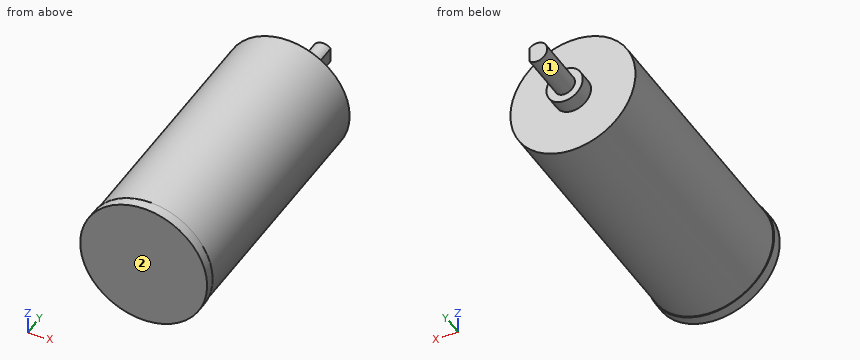
```python
from build123d import *

# Parameters (mm, degrees)
SKETCH_1_R      = 12.25
EXTRUDE_1_DEPTH = 2
SKETCH_2_R      = 12.075
EXTRUDE_2_DEPTH = 51.65
SKETCH_3_R      = 3.5
EXTRUDE_3_DEPTH = 3
EXTRUDE_4_DEPTH = 10


with BuildPart() as part:
    # Эскиз1 → Бобышка-Вытянуть1 (new body)
    with BuildSketch(Plane(origin=(0, 0, 0), x_dir=(1, 0, 0), z_dir=(0, 1, 0))):
        Circle(SKETCH_1_R)
    extrude(amount=EXTRUDE_1_DEPTH)

    # Эскиз2 → Бобышка-Вытянуть2 (add)
    with BuildSketch(Plane(origin=(0, 0, 0), x_dir=(1, 0, 0), z_dir=(0, 1, 0))):
        Circle(SKETCH_2_R)
    extrude(amount=EXTRUDE_2_DEPTH)

    # Эскиз3 → Бобышка-Вытянуть3 (add)
    with BuildSketch(Plane(origin=(0, 51.65, 0), x_dir=(1, 0, 0), z_dir=(0, 1, 0))):
        Circle(SKETCH_3_R)
    extrude(amount=EXTRUDE_3_DEPTH)

    # Эскиз4 → Бобышка-Вытянуть4 (add)
    with BuildSketch(Plane(origin=(0, 54.65, 0), x_dir=(1, 0, 0), z_dir=(0, 1, 0))):
        with BuildLine():
            Line((1.45, 0), (1.45, 1.377497731))
            ThreePointArc((1.45, 1.377497731), (-2, 0), (1.45, -1.377497731))
            Line((1.45, -1.377497731), (1.45, 0))
        make_face()
    extrude(amount=EXTRUDE_4_DEPTH)


solid = part.part
```
For this review, take the finished solid that the model builds, in its own axes (mm). Face numbers are marked on the shaded views. A direction names the side the tool comes from. Coordinates: 2 decimals unless noted, no trailing zeros. Write each loop counter-clockwise with the first axis right and the second up, starting at its lowest first coordinate (ties: lowest second). Pieces come first, ordered by that corner, then holes. Notation, with made-up numbers: (25, 1) - (34, 1) arc R23 ccw to (34, 22) - close; hole circle Ø6 at (37, 17). An arc over 180 degrees is marked (long way). Put each result on its own line as item: value.
1. Add section C-C, the plane y = 29. Give the boundary of the cut face in (x, z) (3 decimals).
Values found:
outline: circle Ø24.15 at (0, 0)
2. For pin 1 (5 mm diameter, centred on y = 9.5, z = -6, fed in from -X); pin 2 (5 mm diameter, centred on x = -3, y = 17.5, fed in from -Z); pin 3 (2 mm diameter, centred on x = 5.5, y = 25, fed in from -Z), all flat-tipped, find the tip position at first contact; note any pin that passes through.
Values found:
pin 1: x = -11.56
pin 2: z = -12.06
pin 3: z = -11.21
3. Wall thickness on probe 1 along Y at (x, z) = (-4.25, -3.5); probe 2 along Z at (x, y) = (-6.5, 41); probe 3 along X at (y, z) = (51, -9): over which ranges is each line inside the solid? List them lowest first.
Values found:
probe 1: 0 to 51.65
probe 2: -10.18 to 10.18
probe 3: -8.05 to 8.05
4. Add section D-D, the plane x = -7. Give the boundary of the cut face in (y, z), then the cut area to 3 significant figures.
Values found:
outline: (0, -10.05) - (2, -10.05) - (2, -9.84) - (51.65, -9.84) - (51.65, 9.84) - (2, 9.84) - (2, 10.05) - (0, 10.05) - close
area: 1,020 mm²
5. Machinability: for the marked faces 1 and 2, which of the approach directions +Z, -Z, +X, -X, +Y, -Y give a long, thin tool a straight path to every point of the face, cutting with its end or side? Answer none if there is none.
Values found:
face 1: +Y
face 2: +Z, -Z, +X, -X, -Y
6. Add section A-A, the plane x = 0. Give the boundary of the cut face in (y, z) (3 decimals).
Values found:
outline: (0, -12.25) - (2, -12.25) - (2, -12.075) - (51.65, -12.075) - (51.65, -3.5) - (54.65, -3.5) - (54.65, -2) - (64.65, -2) - (64.65, 2) - (54.65, 2) - (54.65, 3.5) - (51.65, 3.5) - (51.65, 12.075) - (2, 12.075) - (2, 12.25) - (0, 12.25) - close
7. Add section B-B, the plane z = 0. Give the boundary of the cut face in (x, y) (3 decimals), then the cut area to 3 significant figures.
Values found:
outline: (-12.25, 0) - (12.25, 0) - (12.25, 2) - (12.075, 2) - (12.075, 51.65) - (3.5, 51.65) - (3.5, 54.65) - (1.45, 54.65) - (1.45, 64.65) - (-2, 64.65) - (-2, 54.65) - (-3.5, 54.65) - (-3.5, 51.65) - (-12.075, 51.65) - (-12.075, 2) - (-12.25, 2) - close
area: 1,300 mm²
